Here's the drawing with two shaded views (mm, measured from the low corner). I have some questions. A direction names the side the tool comes from. Give positions to 0.01 mm unless a question says otherwise; leave off trailing zeros. Write each loop counter-clockwise with the first axis right and the second up, starting at its lowest first coordinate (ties: lowest second). Pieces come first, ordered by that corner, then holes.
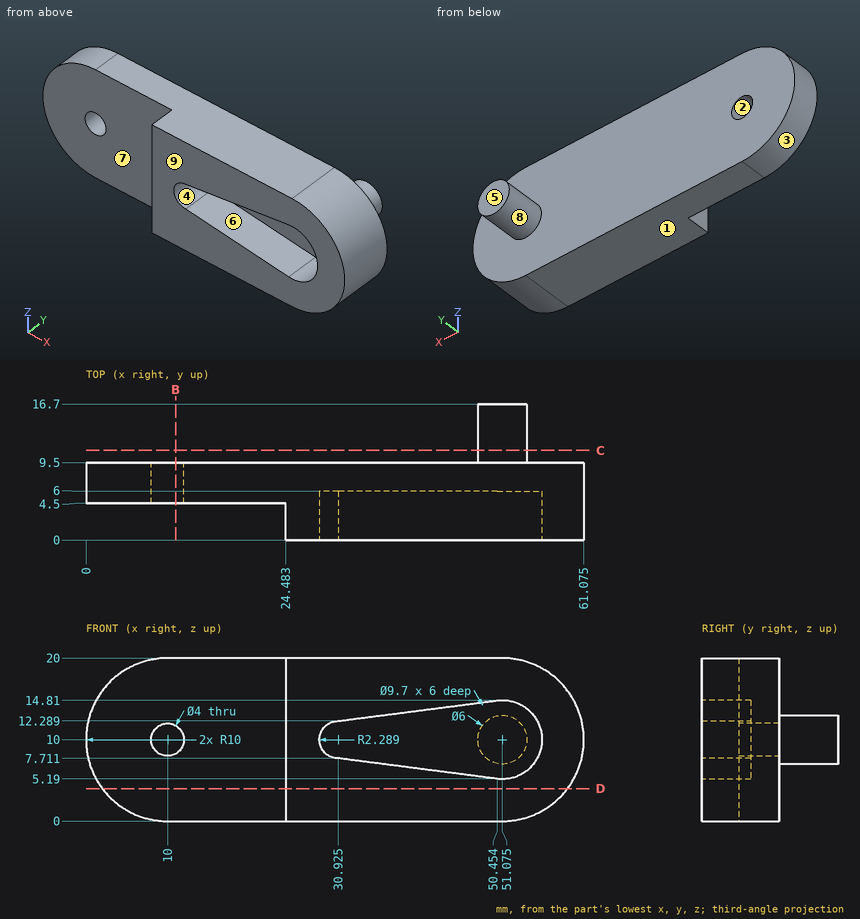
(1) Imagine slicing it at C-C, the plane y = 11. Write out the boundary of the cut face in (x, z) (1 decimal), plus the area to 3 significant figures.
Returned:
outline: circle Ø6 at (51.1, 10)
area: 28.3 mm2
(2) Will these pins go through, and if not, where does the flat tip stop? P1, Ø6, axis at x = 33, z = 5.5, coming from the +Y side; P2, Ø2, axis at y = 2.5, z = 9.5, coming from the -X side; P3, Ø3, axis at x = 50.5, z = 7, coming from the +Y side; P4, Ø5, axis at y = 6, z = 5.5, coming from the +X side.
Returned:
P1: stops at y = 9.5
P2: stops at x = 24.48
P3: stops at y = 16.7
P4: stops at x = 60.87
(3) For the marked faces 5, 6, 7, 8 and 9, which set-ups out of +Z, -Z, +X, -X, +Y, -Y let a thin tool reach every point of the face, with its end or its side?
Returned:
face 5: +Z, -Z, +X, -X, +Y
face 6: -Y
face 7: +Z, -Z, -X, -Y
face 8: +Y
face 9: +Z, -Z, +X, -X, -Y
(4) Imagine slicing it at B-B, the plane x = 11. Write out the boundary of the cut face in (y, z).
Returned:
outline: (4.5, 0) - (9.5, 0) - (9.5, 8.27) - (4.5, 8.27) - close; (4.5, 11.73) - (9.5, 11.73) - (9.5, 20) - (4.5, 20) - close
(5) If we mould it in two halves opening along Z, with no side actions, what happens to the marked faces 1, 2, 3 and 4? For each: +Z half, -Z half, draft (parallel to the pull), parting line (faces both ways), or undercut.
Returned:
face 1: -Z half
face 2: undercut
face 3: parting line
face 4: undercut
(6) Imagine slicing it at D-D, the plane z = 4. Write out the boundary of the cut face in (x, y) (1 decimal), plus the area to 3 significant figures.
Returned:
outline: (2, 4.5) - (24.5, 4.5) - (24.5, 0) - (59.1, 0) - (59.1, 9.5) - (2, 9.5) - close
area: 441 mm2
(7) If I drill on L1, parallel to X at y = 1.3, z = 10 (1 decimal); L2, parallel to X at y = 6.8, z = 10 (1 decimal); L3, parallel to Y at x = 35.5, z = 8.25, over which ranges is the centre line in solid material (lowest first)?
Returned:
L1: x = 24.5 to 28.6, 55.9 to 61.1
L2: x = 0 to 8, 12 to 61.1
L3: y = 6 to 9.5
